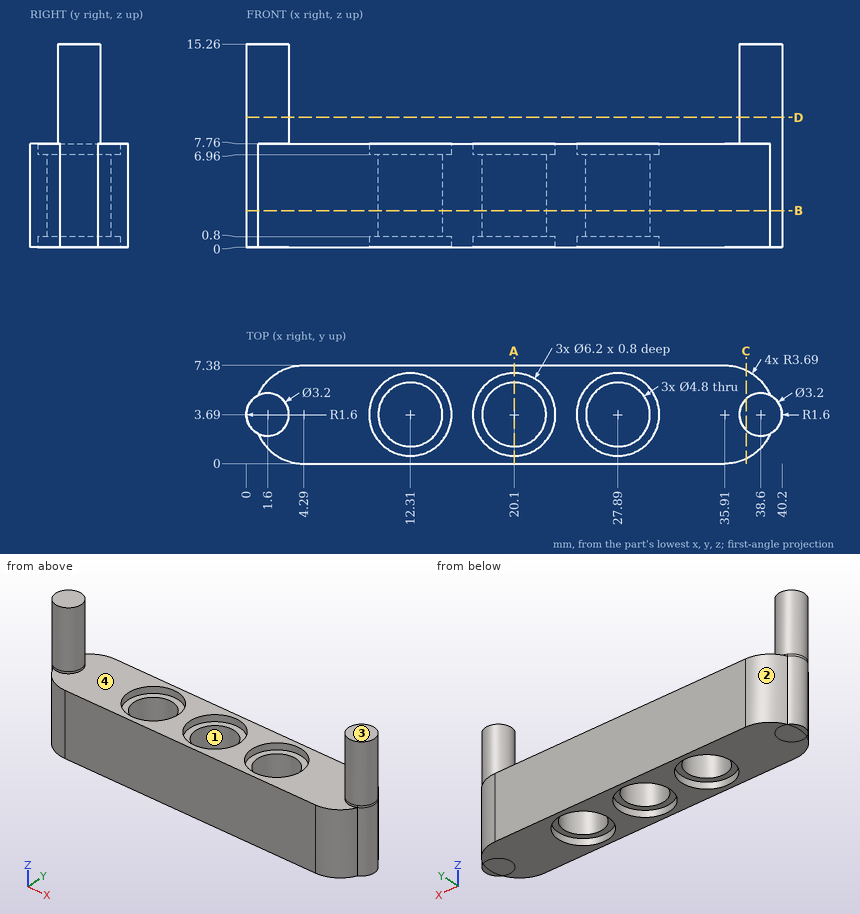
Input: dimensioned drawing with shaded views. Units: mm. Origin: part minimum x, y, z. Give positions to 0.01 mm unless a question says otherwise; leave off trailing zeros. Order: outer loops, then holes, each group sorted by start corner. A loop starts at its lowest first (then second) coordinate and runs counter-clockwise, first axis right, second up. Notation, with made-up numbers: (-40, 73.5) -> (15, 73.5) arc R31 cw to (15, 104.5) -> close; hole circle Ø6 at (66.25, 28.5). An arc over 180 degrees is marked (long way). Use one line per item in the form item = value.
1) Section D-D, the plane z = 9.75. Return loops of the section in (x, y), and give its area (3 significant figures).
Response values:
outline = circle Ø3.2 at (1.6, 3.69); circle Ø3.2 at (38.6, 3.69)
area = 16.1 mm^2
2) Line query: probe 1 along Y at (x, z) = (27.89, 5.75); probe 2 along X at (y, z) = (3.75, 14.5); probe 3 along Y at (x, z) = (38.5, 9). Output: solid intervals per line, ascending.
Response values:
probe_1 = 0 to 1.29, 6.09 to 7.38
probe_2 = 0 to 3.2, 37 to 40.2
probe_3 = 2.09 to 5.29
3) Mould query, pull axis X, two halves, no side actions, for the marked faces 1, 2, 3 and 4. Classes: pulls with the +X half, pulls with the -X half, needs draft (parallel to the pull), parting line crosses it, or undercut.
Response values:
face_1 = undercut
face_2 = pulls with the -X half
face_3 = needs draft
face_4 = undercut
4) Section A-A, the plane x = 20.1. Return loops of the section in (y, z).
Response values:
outline = (0, 0) -> (0.59, 0) -> (0.59, 0.8) -> (1.29, 0.8) -> (1.29, 6.96) -> (0.59, 6.96) -> (0.59, 7.76) -> (0, 7.76) -> close; (6.09, 0.8) -> (6.79, 0.8) -> (6.79, 0) -> (7.38, 0) -> (7.38, 7.76) -> (6.79, 7.76) -> (6.79, 6.96) -> (6.09, 6.96) -> close
5) First-contact query: pin 1 Ø1.5 at (x, y) = (7, 6.5) entering from +Z; pin 2 Ø3 at (x, y) = (27, 2.5) entering from +Z. Flat tips, straight axial feed; report the tip coordinate or a pass-through.
Response values:
pin_1 = 7.76
pin_2 = 6.96
6) Section C-C, the plane x = 37.5. Return loops of the section in (y, z), and give its area (3 significant figures).
Response values:
outline = (0.36, 0) -> (7.02, 0) -> (7.02, 7.76) -> (4.85, 7.76) -> (4.85, 15.26) -> (2.53, 15.26) -> (2.53, 7.76) -> (0.36, 7.76) -> close
area = 69.1 mm^2
7) Section B-B, the plane z = 2.75. Return loops of the section in (x, y).
Response values:
outline = (0.89, 2.26) arc R3.69 ccw to (4.29, 0) -> (35.91, 0) arc R3.69 ccw to (39.31, 2.26) arc R1.6 ccw to (39.31, 5.12) arc R3.69 ccw to (35.91, 7.38) -> (4.29, 7.38) arc R3.69 ccw to (0.89, 5.12) arc R1.6 ccw to start; hole circle Ø4.8 at (12.31, 3.69); hole circle Ø4.8 at (20.1, 3.69); hole circle Ø4.8 at (27.89, 3.69)
